Can you work these out from the model? Positions are in its coordinate system, mm. Face numbers are marked on the shaded views. A direction names the side the tool comes from. Give positions to 0.01 mm unless a question says otherwise; leave off trailing zeros. Loops run counter-clockwise (first coordinate to the right, second up) from the corner with the lowest first, then second, coordinate; pieces in that order, holes last. Notation, with made-up numbers: M 52.25,15.5 L 67.25,15.5 A21 cw 67.25,35.5 Z; hole C 51.25,-10 d5. An arc over 180 degrees is marked long. Put each result on its own line as item: value. Start each with the question number.
1) Please list where these lines run through material, in increasing order: line 1 along Z through (x, y) = (-8, 32); line 2 along Y through (x, z) = (-5, -7.5); line 3 along Y through (x, z) = (-4, 12). Write a range as from..to.
2) Imagine slicing it at A-A (y = 11). Write out the boundary of the cut face in (x, z), then the cut area to 3 significant figures.
3) Imagine slicing it at B-B (y = 32.5). Write out the boundary of the cut face in (x, z), then the cut area to 3 significant figures.
4) For the marked faces 5, 6 and 7, which set-ups out of +Z, -Z, +X, -X, +Y, -Y let a thin tool reach every point of the face, with its end or its side?
5) For P1, Ø5, axis at x = -1, z = 20, coming from the +Y side; P2, Ø21, axis at y = 26.5, z = -0.5, coming from the -X side; P3, Ø11.5, axis at x = 11.5, z = -4.5, coming from the +Y side; P4, Ø10, axis at y = 32.5, z = 12.5, coming from the -X side, each with a flat end and sliding along its axis, tell me the tip position at first contact or that it passes through.
6) Imagine slicing it at D-D (y = 38.5). Write out the boundary of the cut face in (x, z), then the cut area to 3 significant figures.
7) If we mould it in two halves opening along Y, with no side actions, what happens to the marked faces 1, 2, 3 and 4? For each: +Y half, -Y half, draft (parallel to the pull), parting line (faces both ways), or undercut.
from build123d import *

# Parameters (mm, degrees)
BOSS_EXTRUDE1_DEPTH = 13.5
SKETCH2_R           = 20.25
BOSS_EXTRUDE2_DEPTH = 5
FILLET1_R           = 2
SKETCH3_R           = 9
SKETCH3_R_2         = 8.5
BOSS_EXTRUDE3_DEPTH = 10


with BuildPart() as part:
    # Sketch1 → Boss-Extrude1 (new body)
    with BuildSketch(Plane(origin=(0, 0, 0), x_dir=(1, 0, 0), z_dir=(0, 1, 0))):
        with BuildLine():
            Line((-9.5, -18.474644787), (-9.5, -22.8))
            ThreePointArc((-9.5, -22.8), (-9.207106781, -23.507106781), (-8.5, -23.8))
            Line((-8.5, -23.8), (8.5, -23.8))
            ThreePointArc((8.5, -23.8), (9.207106781, -23.507106781), (9.5, -22.8))
            Line((9.5, -22.8), (9.5, -18.474644787))
            ThreePointArc((9.5, -18.474644787), (9.635674353, -17.97171221), (10.005882353, -17.605249738))
            ThreePointArc((10.005882353, -17.605249738), (0, 20.25), (-10.005882353, -17.605249738))
            ThreePointArc((-10.005882353, -17.605249738), (-9.635674353, -17.97171221), (-9.5, -18.474644787))
        make_face()
    extrude(amount=BOSS_EXTRUDE1_DEPTH)

    # Sketch2 → Boss-Extrude2 (add)
    with BuildSketch(Plane(origin=(0, 13.5, 0), x_dir=(1, 0, 0), z_dir=(0, 1, 0))):
        with Locations(Location((0, 0, 0), (0, 0, 90))):
            Circle(SKETCH2_R)
    extrude(amount=BOSS_EXTRUDE2_DEPTH)

    # Fillet1
    fillet1_edges = [part.edges().sort_by_distance(p)[0] for p in [
        (0, 18.5, 20.25),
    ]]
    fillet(fillet1_edges, radius=FILLET1_R)

    # Sketch3 → Boss-Extrude3 (add)
    with BuildSketch(Plane(origin=(0, 0, 0), x_dir=(0, 0, -1), z_dir=(1, 0, 0))):
        with BuildLine():
            Line((17.5, 18.5), (17.5, 22.5))
            ThreePointArc((17.5, 22.5), (17.153602274, 24.396242961), (17.734313483, 26.234313483))
            ThreePointArc((17.734313483, 26.234313483), (15.290492633, 41.627333923), (-0.2953125, 41.6232178))
            ThreePointArc((-0.2953125, 41.6232178), (-2.816482529, 40.665036752), (-5.372782258, 41.525118684))
            ThreePointArc((-5.372782258, 41.525118684), (-21.696710883, 39.404383313), (-19.177419355, 23.137197494))
            ThreePointArc((-19.177419355, 23.137197494), (-17.943996444, 21.712192415), (-17.5, 19.880570536))
            Line((-17.5, 19.880570536), (-17.5, 18.5))
            Line((-17.5, 18.5), (17.5, 18.5))
        make_face()
        with Locations((7.5, 32.5)):
            Circle(SKETCH3_R, mode=Mode.SUBTRACT)
        with Locations((-12.5, 32.5)):
            Circle(SKETCH3_R_2, mode=Mode.SUBTRACT)
    extrude(amount=-BOSS_EXTRUDE3_DEPTH)


solid = part.part
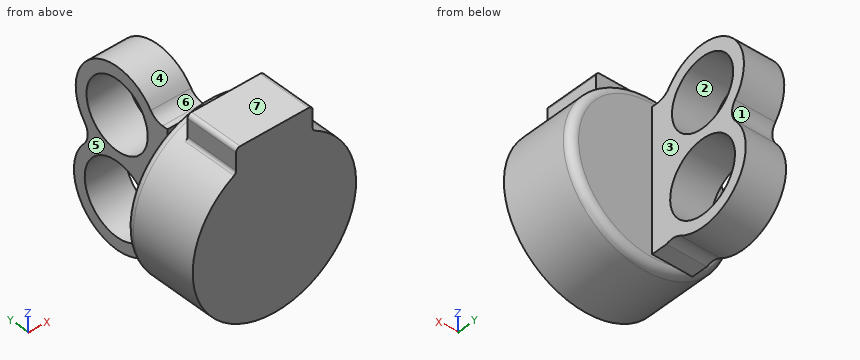
Recorded:
1. line 1: -19.49..-16.49, 1.49..4.01, 20.99..23.99
1. line 2: 0..23.5, 41.5..44.5
1. line 3: 0..24.01, 40.99..43.99
2. outline: M -10.01,17.61 A20.25 ccw long 10.01,17.61 A1 cw 9.5,18.47 L 9.5,22.8 A1 ccw 8.5,23.8 L -8.5,23.8 A1 ccw -9.5,22.8 L -9.5,18.47 A1 cw Z
2. area: 1,370 mm²
3. outline: M -10,-19.5 L 0,-19.5 L 0,-16.5 L -10,-16.5 Z; M -10,1.5 L 0,1.5 L 0,4 L -10,4 Z; M -10,21 L 0,21 L 0,24 L -10,24 Z
3. area: 85.0 mm²
4. face 5: +Z, -Z, -X, +Y
4. face 6: +Z, +X, -X
4. face 7: +Z, +X, -X, -Y
5. P1: y = 42.86
5. P2: x = -20.25
5. P3: y = 18.5
5. P4: through
6. outline: M -10,-17.89 L 0,-17.89 L 0,-14.21 L -10,-14.21 Z; M -10,-0.79 L 0,-0.79 L 0,6.48 L -10,6.48 Z; M -10,18.52 L 0,18.52 L 0,22.31 L -10,22.31 Z
6. area: 147 mm²
7. face 1: +Y half
7. face 2: undercut
7. face 3: draft
7. face 4: undercut
